Input: part model. Units: mm. Frame: model coordinates. Face numbers are marked on the shaded views. A direction names the side the tool comes from. Coordinates: 2 decimals unless noted, no trailing zeros. Order: outer loops, then holes, each group sorted by start corner. A loop starts at its lowest first (then second) coordinate and runs counter-clockwise, first axis right, second up. Notation, with made-up numbers: (-8, -12.75) -> (50, -12.75) arc R16 ccw to (50, -1.75) -> close; hole circle Ø9 at (49, 75). An arc over 180 degrees is marked (long way). Use one line per item in the form item = value. Start each with the question number.
1) Section query A-A on x = 7. Output: boundary loops of the cut face in (y, z), then the cut area to 3 significant figures.
2) Access query for the marked faces 1, 2, 3, 4 and 5. Directions: +Z, -Z, +X, -X, +Y, -Y. A direction counts if a zero-diameter tool reaches every point of the face in a straight line with its end or side. Return the directions, or none.
3) Ray query, line 1 along Y through (x, z) = (8.5, 86). Return the intervals inside material, ascending.
4) Section query C-C on z = 92. Output: boundary loops of the cut face in (x, y).
5) Section query B-B on y = 72. Output: boundary loops of the cut face in (x, z).
6) Pin query (flat end, axial travel): pin 1 (3 mm diameter, centred on x = 4.5, z = 25.5, fed in from -Y); pin 2 (5 mm diameter, centred on y = 24.5, z = 87, fed in from -X); pin 3 (3 mm diameter, centred on x = 4.5, z = 92, fed in from +Y); pin 4 (5 mm diameter, centred on x = 6.5, y = 6.5, fed in from -Z). Return the tip coordinate at first contact, or that it passes through.
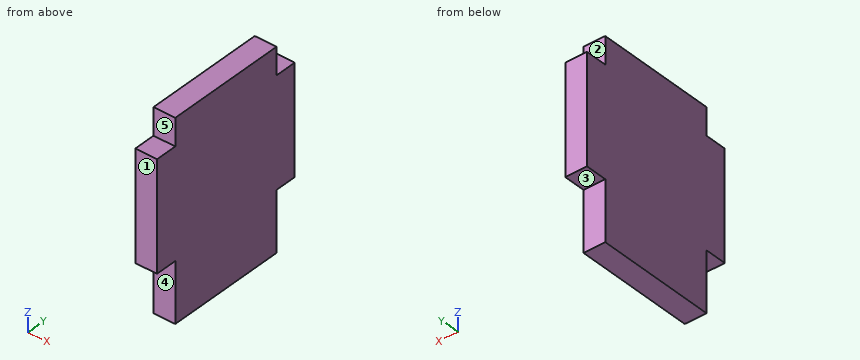
Autodesk Inventor part; units mm, degrees
ref_plane "YZ Plane" through (0, 0, 0) normal (1, 0, 0) x (0, 1, 0)
ref_plane "XZ Plane" through (0, 0, 0) normal (0, 1, 0) x (-1, 0, 0)
ref_plane "XY Plane" through (0, 0, 0) normal (0, 0, 1) x (1, 0, 0)
sketch "Sketch1" plane through (0, 0, 0) normal (1, 0, 0) x (0, 1, 0)
  line L0 (69.0933, 8.2135) -> (13.6933, 8.2135)
  line L1 (13.6933, 8.2135) -> (13.6933, 35.7135)
  line L2 (13.6933, 35.7135) -> (3.6933, 35.7135)
  line L3 (3.6933, 35.7135) -> (3.6933, 85.7135)
  line L4 (3.6933, 85.7135) -> (13.6933, 85.7135)
  line L5 (13.6933, 85.7135) -> (13.6933, 98.2135)
  line L6 (13.6933, 98.2135) -> (69.0933, 98.2135)
  line L7 (69.0933, 98.2135) -> (69.0933, 85.7135)
  line L8 (69.0933, 85.7135) -> (79.0933, 85.7135)
  line L9 (79.0933, 85.7135) -> (79.0933, 35.7135)
  line L10 (79.0933, 35.7135) -> (69.0933, 35.7135)
  line L11 (69.0933, 35.7135) -> (69.0933, 8.2135)
  point P0 (0, 0)
  dimension "d0" = 55.4
  dimension "d1" = 10
  dimension "d2" = 10
  dimension "d3" = 10
  dimension "d4" = 27.5
  dimension "d5" = 12.5
  dimension "d8" = 50
extrude "Extrusion1" add sketch "Sketch1" along normal blind 10
equation "\"d1\" = Width"
equation "\"d2\" = Width"
equation "\"d3\" = Width"
equation "\"d6\" = Width"
equation "\"Width\" = 10"
properties part number "SideWall" material "ABS Plastic"
Answers below:
q1.outline = (3.69, 35.71) -> (13.69, 35.71) -> (13.69, 8.21) -> (69.09, 8.21) -> (69.09, 35.71) -> (79.09, 35.71) -> (79.09, 85.71) -> (69.09, 85.71) -> (69.09, 98.21) -> (13.69, 98.21) -> (13.69, 85.71) -> (3.69, 85.71) -> close
q1.area = 5,990 mm^2
q2.face_1 = +Z, -Z, +X, -X, -Y
q2.face_2 = +Z, +X, -X, +Y
q2.face_3 = -Z, +X, -X, +Y
q2.face_4 = -Z, +X, -X, -Y
q2.face_5 = +Z, +X, -X, -Y
q3.line_1 = 13.69 to 69.09
q4.outline = (0, 13.69) -> (10, 13.69) -> (10, 69.09) -> (0, 69.09) -> close
q5.outline = (0, 35.71) -> (10, 35.71) -> (10, 85.71) -> (0, 85.71) -> close
q6.pin_1 = 13.69
q6.pin_2 = 0
q6.pin_3 = 69.09
q6.pin_4 = 35.71
